Could you check a few things on this model? Use its own coordinates, in mm. Give positions to 0.01 mm unless a question says otherwise; leave off trailing zeros. Loops run counter-clockwise (first coordinate to the right, second up) from the corner with the lowest first, then second, coordinate; pieces in that order, holes last. Notation, with made-up numbers: M -31,84.25 L -24,84.25 A14 cw -24,88.25 Z; hole C 18,82.5 d10. An arc over 180 degrees is marked long. Use CSV: the item, a comma, the result in double quotes.
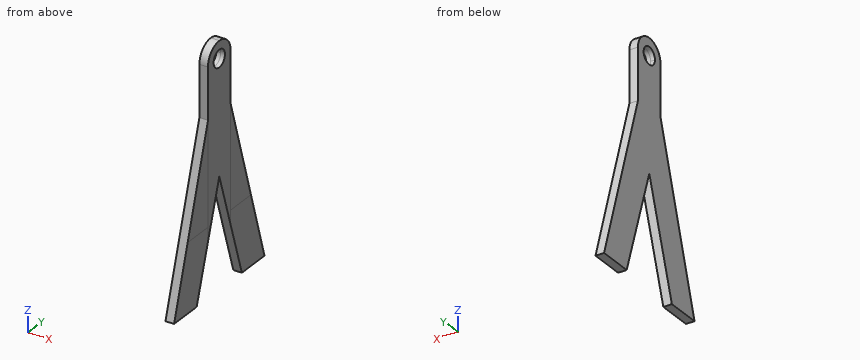
```python
from build123d import *

# Parameters (mm, degrees)
F0_W        = 6.35
F0_H        = 25.4
F1_DEPTH    = 177.8
F0_H_2      = 38.1
F2_DEPTH    = 50.8
F4_D        = 12.7
F4_DEPTH    = 3.176
F5_D        = 12.7
F6_R        = 12.69999
F7_DEPTH    = 127
F8_T4_DEPTH = 665.7191836207
F8_T9_DEPTH = 665.7191836207
F11_DEPTH   = 25.4


# Not quite as in the source:
# - a fillet or chamfer that OpenCascade refuses, or shapes differently, is made with other operations: its cross-section is extruded or revolved along the edge and cut away or added
# - two fillets or chamfers of one size are made in one step
# - a fillet or chamfer is up to 0.001 mm smaller than in the source, because OpenCascade refuses the exact size


with BuildPart() as f1:
    # F0 (on Top) → F1 (new body)
    with BuildSketch(Plane.XY):
        Rectangle(F0_W, F0_H)
    extrude(amount=F1_DEPTH)

    # F0 (on Top) → F2 (join)
    with BuildSketch(Plane.XY):
        with Locations((0, 31.75)):
            Rectangle(F0_W, F0_H_2)
        with Locations((0, -31.75)):
            Rectangle(F0_W, F0_H_2)
    extrude(amount=F2_DEPTH)

    # F4 (through all, one way)
    with BuildSketch(Plane.YZ):
        with Locations((0, 165.1)):
            Circle(F4_D / 2)
    extrude(amount=-F4_DEPTH, mode=Mode.SUBTRACT)

    # F5 (through all)
    with Locations(Plane(origin=(0, 0, 0), x_dir=(0, 1, 0), z_dir=(-1, 0, 0))):
        with Locations((0, -165.1)):
            Hole(F5_D / 2)

    # F6 (radius 12.7 in the source; OpenCascade refuses exactly that, so slightly less here)
    f6_edges = [f1.edges().sort_by_distance(p)[0] for p in [
        (0, -12.7, 177.8),
        (0, 12.7, 177.8),
    ]]
    fillet(f6_edges, radius=F6_R)

    # F0 (on Top) → F7 (join)
    with BuildSketch(Plane.XY):
        with Locations((0, -31.75)):
            Rectangle(F0_W, F0_H_2)
        with Locations((0, 31.75)):
            Rectangle(F0_W, F0_H_2)
    extrude(amount=F7_DEPTH)

    # F8: chamfer of 38.1 x 127 on 2 edges, made by hand


with BuildPart() as f8_tool2:
    # F8_s3 → F8_t4 (new body)
    with BuildSketch(Plane.YZ.offset(332.8595918104)):
        Polygon((50.8, 0), (12.7, 127), (50.8, 127), align=None)
    extrude(amount=-F8_T4_DEPTH)

    split(bisect_by=Plane.XZ.offset(-12.7), keep=Keep.BOTTOM)


with BuildPart() as f1_1:
    add(f1.part)

    # F8_t1: cut F8_tool2
    add(f8_tool2.part, mode=Mode.SUBTRACT)


with BuildPart() as f8_tool7:
    # F8_s8 → F8_t9 (new body)
    with BuildSketch(Plane.YZ.offset(-332.8595918104)):
        Polygon((-12.7, 127), (-50.8, 0), (-50.8, 127), align=None)
    extrude(amount=F8_T9_DEPTH)

    split(bisect_by=Plane.XZ.offset(12.7), keep=Keep.TOP)


with BuildPart() as f1_2:
    add(f1_1.part)

    # F8_t6: cut F8_tool7
    add(f8_tool7.part, mode=Mode.SUBTRACT)

    # F10 (on face) → F11 (cut)
    with BuildSketch(Plane.YZ.offset(3.175)):
        Polygon((25.4, 0), (0, 80.9457584765), (-25.4, 0), align=None)
    extrude(amount=-F11_DEPTH, mode=Mode.SUBTRACT)


solid = f1_2.part
```
1. I want a section at A-A, the plane z = 20.5. List the corners of the cut face in (x, y) for me (3 decimals), then the cut area to 3 significant figures.
Outcome:
outline,"M -3.175,-44.65 L 3.175,-44.65 L 3.175,-18.967 L -3.175,-18.967 Z; M -3.175,18.967 L 3.175,18.967 L 3.175,44.65 L -3.175,44.65 Z"
area,"326 mm2"
2. I want a section at C-C, the plane y = 32.5. List the corners of the cut face in (x, z) for me (3 decimals).
Outcome:
outline,"M -3.175,0 L 3.175,0 L 3.175,61 L -3.175,61 Z"
3. I want a section at D-D, the plane z = 115.5. List the corners of the cut face in (x, y) for me (3 decimals).
Outcome:
outline,"M -3.175,-16.15 L 3.175,-16.15 L 3.175,16.15 L -3.175,16.15 Z"
4. I'm going to push flat-ended pins straight in: pin 1 Ø1.5 at (x, z) = (-1.5, 47) entering from +Y (3 decimals); pin 2 Ø3 at (x, z) = (1, 147.5) entering from +Y. Where does each tip first touch, or does it pass through?
Outcome:
pin 1,"y = 36.925"
pin 2,"y = 12.7"
5. Please list where these lines run through material, in increasing order: line 1 (Y direction, x = 1.5, z = 165.1); line 2 (Y direction, x = 0.5, z = 147.5); line 3 (Y direction, x = -3, z = 39).
Outcome:
line 1,"-12.7 to -6.35, 6.35 to 12.7"
line 2,"-12.7 to 12.7"
line 3,"-39.1 to -13.16, 13.16 to 39.1"
